Geometry check sheet. Reference: the model listing, model coordinates, mm. A direction names the side the tool comes from. Round coordinates to 2 decimals unless told otherwise and drop trailing zeros. Order: outer loops, then holes, each group sorted by start corner. A loop starts at its lowest first (then second) coordinate and runs counter-clockwise, first axis right, second up. Notation, with made-up numbers: (38.5, 60.25) -> (87.5, 60.25) arc R22 ccw to (87.5, 97.25) -> close; hole circle Ø5 at (77.5, 75). An arc over 180 degrees is marked (long way). Answer as a JSON object with one key per item and string values. Group by question number.
Autodesk Inventor part; units mm, degrees
ref_plane "YZ Plane" through (0, 0, 0) normal (1, 0, 0) x (0, 1, 0)
ref_plane "XZ Plane" through (0, 0, 0) normal (0, 1, 0) x (-1, 0, 0)
ref_plane "XY Plane" through (0, 0, 0) normal (0, 0, 1) x (1, 0, 0)
sketch "Sketch1" plane through (0, 0, 0) normal (1, 0, 0) x (0, 1, 0)
  line L0 (41, 41) -> (-41, 41)
  line L1 (-41, 41) -> (-41, -41)
  line L2 (-41, -41) -> (41, -41)
  line L3 (41, -41) -> (41, 41)
  point P0 (0, 0)
  point P1 (0, 41)
  point P2 (41, 0)
  dimension "d0" = 82
  dimension "d1" = 82
extrude "Extrusion1" add sketch "Sketch1" along normal mid plane 2
sketch "Sketch2" plane through (-1, 0, 0) normal (-1, 0, 0) x (0, 0, 1)
  line L0 (31.6667, 22) -> (37, 26)
  arc A0 (25.6667, 20) -> (31.6667, 22) centre (25.6667, 30) ccw
  line L1 (17.5, 20) -> (25.6667, 20)
  line L2 (17.5, 20) -> (17.5, 18.2355)
  line L3 (-17.5, 18.2356) -> (17.5, 18.2356)
  line L4 (-17.5, 20) -> (-17.5, 18.2355)
  line L5 (-25.6667, 20) -> (-17.5, 20)
  arc A1 (-31.6667, 22) -> (-25.6667, 20) centre (-25.6667, 30) ccw
  line L6 (-37, 26) -> (-31.6667, 22)
  arc A2 (-41, 34) -> (-37, 26) centre (-31, 34) ccw
  line L7 (-41, 37) -> (-41, 34)
  arc A3 (-37, 41) -> (-41, 37) centre (-37, 37) ccw
  line L8 (-37, 41) -> (-25.3705, 41)
  arc A4 (-18.9687, 38.6822) -> (-25.3705, 41) centre (-25.3705, 31) ccw
  line L9 (-18.9687, 38.6822) -> (-12.5313, 33.3178)
  arc A5 (-12.5313, 33.3178) -> (-6.1295, 31) centre (-6.1295, 41) ccw
  line L10 (-6.1295, 31) -> (6.1295, 31)
  arc A6 (6.1295, 31) -> (12.5313, 33.3178) centre (6.1295, 41) ccw
  line L11 (12.5313, 33.3178) -> (18.9687, 38.6822)
  arc A7 (25.3705, 41) -> (18.9687, 38.6822) centre (25.3705, 31) ccw
  line L12 (25.3705, 41) -> (37, 41)
  arc A8 (41, 37) -> (37, 41) centre (37, 37) ccw
  line L13 (41, 37) -> (41, 34)
  arc A9 (37, 26) -> (41, 34) centre (31, 34) ccw
  circle A10 centre (36, 36.9) radius 1.35
  circle A11 centre (-36, 36.9) radius 1.35
  line L14 (-25.6667, 20) -> (-25.6667, 5)
  line L15 (25.6667, 20) -> (25.6667, 5)
  line L16 (25.6667, 5) -> (-25.6667, 5)
  point P0 (0, 0)
  dimension "d4" = 15
extrude "Extrusion2" add sketch "Sketch2" along normal blind 2
sketch "Sketch3" plane through (1, 0, 0) normal (1, 0, 0) x (0, 0, -1)
  line L0 (-31.6667, 22) -> (-37, 26)
  arc A0 (-41, 34) -> (-37, 26) centre (-31, 34) ccw
  line L1 (-41, 34) -> (-41, 37)
  arc A1 (-37, 41) -> (-41, 37) centre (-37, 37) ccw
  line L2 (-37, 41) -> (-25.3705, 41)
  arc A2 (-18.9687, 38.6822) -> (-25.3705, 41) centre (-25.3705, 31) ccw
  line L3 (-18.9687, 38.6822) -> (-12.5313, 33.3178)
  arc A3 (-12.5313, 33.3178) -> (-6.1295, 31) centre (-6.1295, 41) ccw
  line L4 (-6.1295, 31) -> (6.1295, 31)
  arc A4 (6.1295, 31) -> (12.5313, 33.3178) centre (6.1295, 41) ccw
  line L5 (12.5313, 33.3178) -> (18.9687, 38.6822)
  arc A5 (25.3705, 41) -> (18.9687, 38.6822) centre (25.3705, 31) ccw
  line L6 (25.3705, 41) -> (37, 41)
  arc A6 (41, 37) -> (37, 41) centre (37, 37) ccw
  line L7 (41, 37) -> (41, 34)
  arc A7 (37, 26) -> (41, 34) centre (31, 34) ccw
  line L8 (37, 26) -> (31.6667, 22)
  arc A8 (25.6667, 20) -> (31.6667, 22) centre (25.6667, 30) ccw
  line L9 (25.6667, 20) -> (25.6667, 5)
  line L10 (25.6667, 5) -> (-25.6667, 5)
  line L11 (-25.6667, 5) -> (-25.6667, 20)
  arc A9 (-31.6667, 22) -> (-25.6667, 20) centre (-25.6667, 30) ccw
  circle A10 centre (-36, 36.9) radius 1.35
  circle A11 centre (36, 36.9) radius 1.35
  line L12 (-41, -41) -> (41, -41)
  line L13 (41, -41) -> (41, 41)
  line L14 (41, 41) -> (-41, 41)
  line L15 (-41, 41) -> (-41, -41)
  point P0 (0, 0)
  point P1 (41, 37)
  point P2 (-37, 41)
  point P3 (25.3705, 41)
  point P4 (-41, 34)
extrude "Extrusion3" cut sketch "Sketch3" against normal blind 15 contours A9 L11 L10 L9 A8 L8 A7 L13 L12 L15 A0 L0 | L15 L14 A1 | L14 A5 L5 A4 L4 A3 L3 A2 | A6 L14 L13
sketch "Sketch4" plane through (-3, 0, 0) normal (-1, 0, 0) x (0, 0, 1)
  line L0 (31.6667, 22) -> (37, 26)
  arc A0 (37, 26) -> (41, 34) centre (31, 34) ccw
  line L1 (41, 34) -> (41, 37)
  arc A1 (41, 37) -> (37, 41) centre (37, 37) ccw
  line L2 (37, 41) -> (25.3705, 41)
  arc A2 (25.3705, 41) -> (18.9687, 38.6822) centre (25.3705, 31) ccw
  line L3 (18.9687, 38.6822) -> (12.5313, 33.3178)
  arc A3 (6.1295, 31) -> (12.5313, 33.3178) centre (6.1295, 41) ccw
  line L4 (6.1295, 31) -> (-6.1295, 31)
  arc A4 (-12.5313, 33.3178) -> (-6.1295, 31) centre (-6.1295, 41) ccw
  line L5 (-12.5313, 33.3178) -> (-18.9687, 38.6822)
  arc A5 (-18.9687, 38.6822) -> (-25.3705, 41) centre (-25.3705, 31) ccw
  line L6 (-25.3705, 41) -> (-37, 41)
  arc A6 (-37, 41) -> (-41, 37) centre (-37, 37) ccw
  line L7 (-41, 37) -> (-41, 34)
  arc A7 (-41, 34) -> (-37, 26) centre (-31, 34) ccw
  line L8 (-37, 26) -> (-31.6667, 22)
  arc A8 (-31.6667, 22) -> (-25.6667, 20) centre (-25.6667, 30) ccw
  line L9 (-25.6667, 20) -> (-25.6667, 5)
  line L10 (-25.6667, 5) -> (25.6667, 5)
  line L11 (25.6667, 5) -> (25.6667, 20)
  arc A9 (25.6667, 20) -> (31.6667, 22) centre (25.6667, 30) ccw
  circle A10 centre (36, 36.9) radius 1.35
  circle A11 centre (-36, 36.9) radius 1.35
  circle A12 centre (-36, 36.9) radius 2.3
  circle A13 centre (36, 36.9) radius 2.3
  point P0 (0, 0)
  dimension "d9" = 4.6
  dimension "d10" = 4.6
extrude "Extrusion4" cut sketch "Sketch4" against normal blind 1.4 contours A12 | A13
sketch "Sketch5" plane through (-3, 0, 0) normal (-1, 0, 0) x (0, 0, 1)
  circle A0 centre (36, 36.9) radius 2.3
  circle A1 centre (-36, 36.9) radius 2.3
  line L0 (31.6667, 22) -> (37, 26)
  arc A2 (37, 26) -> (41, 34) centre (31, 34) ccw
  line L1 (41, 34) -> (41, 37)
  arc A3 (41, 37) -> (37, 41) centre (37, 37) ccw
  line L2 (37, 41) -> (25.3705, 41)
  arc A4 (25.3705, 41) -> (18.9687, 38.6822) centre (25.3705, 31) ccw
  line L3 (18.9687, 38.6822) -> (12.5313, 33.3178)
  arc A5 (6.1295, 31) -> (12.5313, 33.3178) centre (6.1295, 41) ccw
  line L4 (6.1295, 31) -> (-6.1295, 31)
  arc A6 (-12.5313, 33.3178) -> (-6.1295, 31) centre (-6.1295, 41) ccw
  line L5 (-12.5313, 33.3178) -> (-18.9687, 38.6822)
  arc A7 (-18.9687, 38.6822) -> (-25.3705, 41) centre (-25.3705, 31) ccw
  line L6 (-25.3705, 41) -> (-37, 41)
  arc A8 (-37, 41) -> (-41, 37) centre (-37, 37) ccw
  line L7 (-41, 37) -> (-41, 34)
  arc A9 (-41, 34) -> (-37, 26) centre (-31, 34) ccw
  line L8 (-37, 26) -> (-31.6667, 22)
  arc A10 (-31.6667, 22) -> (-25.6667, 20) centre (-25.6667, 30) ccw
  line L9 (-25.6667, 20) -> (-25.6667, 5)
  line L10 (-25.6667, 5) -> (25.6667, 5)
  line L11 (25.6667, 5) -> (25.6667, 20)
  arc A11 (25.6667, 20) -> (31.6667, 22) centre (25.6667, 30) ccw
  circle A12 centre (-36, 36.9) radius 1.3
  circle A13 centre (36, 36.9) radius 1.3
  point P0 (0, 0)
  dimension "d13" = 2.6
  dimension "d14" = 2.6
extrude "Extrusion5" cut sketch "Sketch5" against normal through all contours A12 | A13
sketch "Sketch6" plane through (1, 0, 0) normal (1, 0, 0) x (0, 0, -1)
  arc A0 (-37, 41) -> (-41, 37) centre (-37, 37) ccw
  line L0 (-41, 37) -> (-41, 34)
  arc A1 (-41, 34) -> (-37, 26) centre (-31, 34) ccw
  line L1 (-37, 26) -> (-31.6667, 22)
  arc A2 (-31.6667, 22) -> (-25.6667, 20) centre (-25.6667, 30) ccw
  line L2 (-25.6667, 20) -> (-25.6667, 5)
  line L3 (-25.6667, 5) -> (25.6667, 5)
  line L4 (25.6667, 5) -> (25.6667, 20)
  arc A3 (25.6667, 20) -> (31.6667, 22) centre (25.6667, 30) ccw
  line L5 (31.6667, 22) -> (37, 26)
  arc A4 (37, 26) -> (41, 34) centre (31, 34) ccw
  line L6 (41, 34) -> (41, 37)
  arc A5 (41, 37) -> (37, 41) centre (37, 37) ccw
  line L7 (37, 41) -> (25.3705, 41)
  arc A6 (25.3705, 41) -> (18.9687, 38.6822) centre (25.3705, 31) ccw
  line L8 (18.9687, 38.6822) -> (12.5313, 33.3178)
  arc A7 (6.1295, 31) -> (12.5313, 33.3178) centre (6.1295, 41) ccw
  line L9 (6.1295, 31) -> (-6.1295, 31)
  arc A8 (-12.5313, 33.3178) -> (-6.1295, 31) centre (-6.1295, 41) ccw
  line L10 (-12.5313, 33.3178) -> (-18.9687, 38.6822)
  arc A9 (-18.9687, 38.6822) -> (-25.3705, 41) centre (-25.3705, 31) ccw
  line L11 (-25.3705, 41) -> (-37, 41)
  circle A10 centre (-20, 9.2) radius 2.05
  circle A11 centre (20, 9.2) radius 2.05
  line L12 (-20, 9.2) -> (20, 9.2) construction
  point P0 (0, 0)
  point P1 (0, 31)
  point P2 (0, 9.2)
  dimension "d17" = 4.1
  dimension "d18" = 4.1
  dimension "d19" = 4.2
  dimension "d20" = 40
extrude "Extrusion6" cut sketch "Sketch6" against normal blind 10 contours A10 | A11
fillet "Fillet1" radius 2 4 edges at (-1, 20, -25.6667) (-1, 5, -25.6667) (-1, 5, 25.6667) (-1, 20, 25.6667)
properties part number "Camera_mount"
Item 1: Depth check by flat-ended pin: pin 1 Ø1 at (x, z) = (-1, -0.5) entering from +Y; pin 2 Ø3 at (y, z) = (36.9, -36) entering from -X; pin 3 Ø1.4 at (y, z) = (37, -35.5) entering from -X; pin 4 Ø1.2 at (x, y) = (-1.5, 14.5) entering from -Z. Enter the tip coordinate at first touch or a pass-through.
Item 2: Sectioned sample at A-A, the plane z = 36. Enter the section's corners in (x, y), then the cut area to 3 significant figures.
Item 3: Sectioned sample at B-B, the plane z = -20. Enter the section's corners in (x, y), then the cut area to 3 significant figures.
Item 4: Sectioned sample at C-C, the plane y = 12. Enter the section's corners in (x, z), then the cut area to 3 significant figures.
Item 5: Thickness scan on L1, parallel to Z at x = -1.1, y = 37; L2, parallel to Y at x = -1.95, z = -36; L3, parallel to Z at x = 0.25, y = 17.5. Record the ranges inside material, lowest first.
Item 6: Mould release check, pull along Y, two halves, no side actions. Record for faces 1 (the cylindrical face through (-0.972, 5.57, -25.065)), 2 (the flat face through (-1.6, 37, -34)), 3 (the flat face through (1, 23, 1)), 4 (the cylindrical face through (-1.986, 40.386, 21.921)): pulls with the +Y half, pulls with the -Y half, needs draft (parallel to the pull), parting line crosses it, or undercut.
Item 7: Set-up check for faces 5 (the flat face through (-0.97, 35.96, 15.7)), 6 (the flat face through (-1, 35, -41)), 7 (the flat face through (-1, 13, -25.667)): record each of +Z, -Z, +X, -X, +Y, -Y from which the full face is reachable in a straight line by a thin tool's end or side.
Item 8: Sectioned sample at D-D, the plane z = 10. Enter the section's corners in (x, y), then the cut area to 3 significant figures.
Result:
{
 "1": {"pin 1": "stops at y = 31", "pin 2": "stops at x = -1.6", "pin 3": "passes through", "pin 4": "stops at z = -25.67"},
 "2": {"outline": "(-3, 25.25) -> (1, 25.25) -> (1, 35.6) -> (-1, 35.6) -> (-1, 35.55) -> (-1.6, 35.55) -> (-1.6, 34.6) -> (-3, 34.6) -> close; (-3, 39.2) -> (-1.6, 39.2) -> (-1.6, 38.25) -> (-1, 38.25) -> (-1, 38.2) -> (1, 38.2) -> (1, 41) -> (-3, 41) -> close", "area": "49.7 mm2"},
 "3": {"outline": "(-3, 5) -> (1, 5) -> (1, 7.15) -> (-3, 7.15) -> close; (-3, 11.25) -> (1, 11.25) -> (1, 39.44) -> (-3, 39.44) -> close", "area": "121 mm2"},
 "4": {"outline": "(-3, -25.67) -> (1, -25.67) -> (1, 25.67) -> (-3, 25.67) -> close", "area": "205 mm2"},
 "5": {"L1": "z = -41 to -37.35, -34.65 to -16.95, 16.95 to 34.65, 37.35 to 41", "L2": "y = 25.25 to 34.6, 39.2 to 41", "L3": "z = -25.67 to 25.67"},
 "6": {"face 1": "pulls with the -Y half", "face 2": "undercut", "face 3": "needs draft", "face 4": "pulls with the +Y half"},
 "7": {"face 5": "+X, -X, +Y", "face 6": "-Z, +X, -X, +Y, -Y", "face 7": "-Z, +X, -X, -Y"},
 "8": {"outline": "(-3, 5) -> (1, 5) -> (1, 31.78) -> (-3, 31.78) -> close", "area": "107 mm2"}
}
